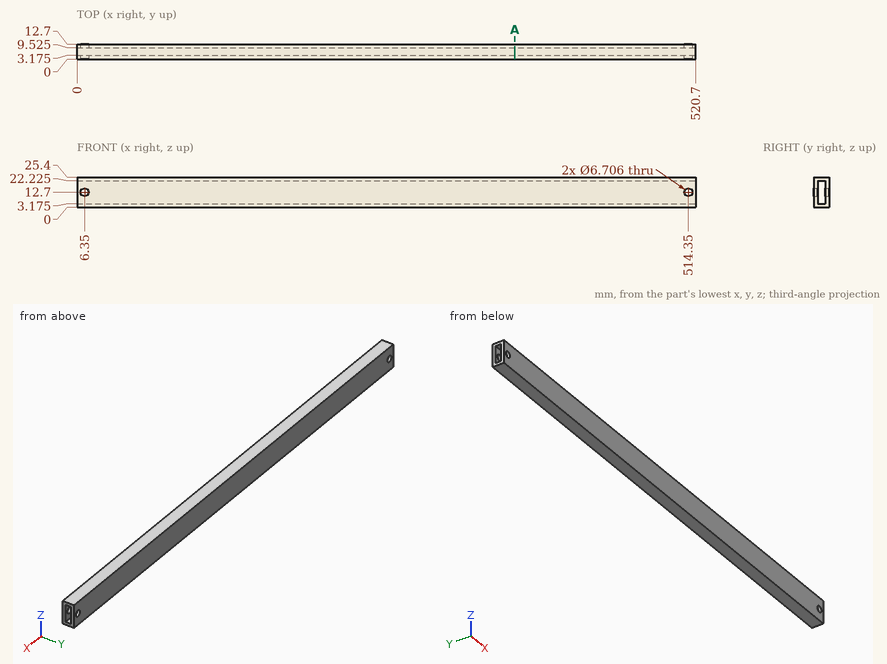
Here's the drawing with two shaded views (mm, measured from the low corner). I have some questions. Give positions to 0.01 mm unless a question says otherwise; leave off trailing zeros. Order: outer loops, then holes, each group sorted by start corner. A loop starts at its lowest first (then second) coordinate and runs counter-clockwise, first axis right, second up. Notation, with made-up numbers: M 77,-13.5 L 127,-13.5 A27 ccw 127,18.5 Z; hole C 67,84 d7. An arc over 180 degrees is marked long. Answer as a JSON object with one key per item and string values. Group by question number.
1) I'm going to push a flat-ended pin straight in: pin 1 Ø6 at (x, z) = (6.35, 12.7) entering from +Y. Where does the tip first touch, or does it pass through?
2) Suppose I cut it at A-A, the plane x = 368.5. Write out the boundary of the cut face in (y, z) (1 decimal), plus the area to 3 significant figures.
3) Please list where these lines run through material, in increasing order: L1, parallel to X at y = 10.35, z = 12.7; L2, parallel to Y at x = 236, z = 14 (1 decimal); L3, parallel to Z at x = 33.5, y = 4.5 (1 decimal). Write a range as [from, to].
Results found:
{
 "1": {"pin 1": "through"},
 "2": {"outline": "M 0,0 L 12.7,0 L 12.7,25.4 L 0,25.4 Z; hole M 3.2,3.2 L 9.5,3.2 L 9.5,22.2 L 3.2,22.2 Z", "area": "202 mm²"},
 "3": {"L1": "[0, 3], [9.7, 511], [517.7, 520.7]", "L2": "[0, 3.2], [9.5, 12.7]", "L3": "[0, 3.2], [22.2, 25.4]"}
}
